```python
from build123d import *

# Parameters (mm, degrees)
BOSS_EXTRUDE1_DEPTH                   = 4
SKETCH3_R                             = 1
CUT_EXTRUDE2_DEPTH                    = 96.498691091
SKETCH4_R                             = 1
CUT_EXTRUDE3_DEPTH                    = 88.017239671
TAP_DRILL_FOR_M3X0_5_TAP2_D           = 2.5
TAP_DRILL_FOR_M3X0_5_TAP2_CSINK_D     = 2.55
TAP_DRILL_FOR_M3X0_5_TAP2_CSINK_ANGLE = 90
M3_CLEARANCE_HOLE2_D                  = 3.6
M3_CLEARANCE_HOLE2_CSINK_D            = 3.65
M3_CLEARANCE_HOLE2_CSINK_ANGLE        = 90
FILLET1_R                             = 2
CHAMFER1_SIZE                         = 2
FILLET2_R                             = 2


# Read off the part's stored shape, not the designer's step: Tap Drill for M3x0.5 Tap4, Tap Drill for M3x0.5 Tap5
with BuildPart() as part:
    # Sketch1 → Boss-Extrude1 (new, symmetric)
    with BuildSketch(Plane(origin=(0, 0, 0), x_dir=(1, 0, 0), z_dir=(0, 1, 0))):
        with BuildLine():
            Line((0, 8), (-10, 8))
            Line((-10, 8), (-10, -8))
            Line((-10, -8), (0, -8))
            Line((0, -8), (0, -14))
            Line((0, -14), (70, -26))
            Line((70, -26), (80, -26))
            Line((80, -26), (80, -20))
            Line((80, -20), (70, -20))
            Line((70, -20), (66.619956187, -19.345797972))
            ThreePointArc((66.619956187, -19.345797972), (65.457260938, -18.655013265), (65, -17.38223827))
            Line((65, -17.38223827), (65, 17.38223827))
            ThreePointArc((65, 17.38223827), (65.457260938, 18.655013265), (66.619956187, 19.345797972))
            Line((66.619956187, 19.345797972), (70, 20))
            Line((70, 20), (80, 20))
            Line((80, 20), (80, 26))
            Line((80, 26), (70, 26))
            Line((70, 26), (0, 14))
            Line((0, 14), (0, 8))
        make_face()
        with BuildLine():
            Line((8, 6.349980206), (8, -6.349980206))
            ThreePointArc((8, -6.349980206), (8.457260938, -7.622755201), (9.619956187, -8.313539907))
            Line((9.619956187, -8.313539907), (54.619956187, -17.023217326))
            ThreePointArc((54.619956187, -17.023217326), (56.272774995, -16.602396687), (57, -15.059657625))
            Line((57, -15.059657625), (57, 15.059657625))
            ThreePointArc((57, 15.059657625), (56.272774995, 16.602396687), (54.619956187, 17.023217326))
            Line((54.619956187, 17.023217326), (9.619956187, 8.313539907))
            ThreePointArc((9.619956187, 8.313539907), (8.457260938, 7.622755201), (8, 6.349980206))
        make_face(mode=Mode.SUBTRACT)
    extrude(amount=BOSS_EXTRUDE1_DEPTH, both=True)

    # Sketch3 → Cut-Extrude2 (cut, through all)
    with BuildSketch(Plane.XY.offset(26)):
        with Locations((75, 0)):
            Circle(SKETCH3_R)
    extrude(amount=-CUT_EXTRUDE2_DEPTH, mode=Mode.SUBTRACT)

    # Sketch4 → Cut-Extrude3 (cut, through all)
    with BuildSketch(Plane.XY.offset(8)):
        with Locations((-7, 0)):
            Circle(SKETCH4_R)
    extrude(amount=-CUT_EXTRUDE3_DEPTH, mode=Mode.SUBTRACT)

    # Tap Drill for M3x0.5 Tap2 (through all)
    with Locations(Plane.XY.offset(8)):
        with Locations((-7, 0)):
            CounterSinkHole(TAP_DRILL_FOR_M3X0_5_TAP2_D / 2, TAP_DRILL_FOR_M3X0_5_TAP2_CSINK_D / 2, counter_sink_angle=TAP_DRILL_FOR_M3X0_5_TAP2_CSINK_ANGLE)

    # M3 Clearance Hole2 (through all)
    with Locations(Plane.XY.offset(26)):
        with Locations((75, 0)):
            CounterSinkHole(M3_CLEARANCE_HOLE2_D / 2, M3_CLEARANCE_HOLE2_CSINK_D / 2, counter_sink_angle=M3_CLEARANCE_HOLE2_CSINK_ANGLE)

    # Fillet1
    fillet1_edges = [part.edges().sort_by_distance(p)[0] for p in [
        (-10, 4, 0),
        (80, -4, -23),
        (80, -4, 23),
        (-10, -4, 0),
        (80, 4, 23),
        (80, 4, -23),
    ]]
    fillet(fillet1_edges, radius=FILLET1_R)

    # Chamfer1
    chamfer1_edges = [part.edges().sort_by_distance(p)[0] for p in [
        (0, 4, 11),
        (0, -4, 11),
        (0, -4, -11),
        (0, 4, -11),
    ]]
    chamfer(chamfer1_edges, length=CHAMFER1_SIZE)

    # Tap Drill for M3x0.5 Tap4 outline → Tap Drill for M3x0.5 Tap4 (revolve, cut)
    with BuildSketch(Plane(origin=(41.33148295, 0, 7.085397077), x_dir=(0.9856222548132666, 0, 0.1689638151108459), z_dir=(0, 1, 0))):
        Polygon((1.25, -13.773711567), (1.25, -7.206179724), (0, -7.206179724), (0, -13.798711567), (1.275, -13.798711567), align=None)
    revolve(axis=Axis((41.33148295, 0, 7.085397077), (0.1689638151108459, 0, -0.9856222548132666)), mode=Mode.SUBTRACT)

    # Tap Drill for M3x0.5 Tap5 outline → Tap Drill for M3x0.5 Tap5 (revolve, cut)
    with BuildSketch(Plane(origin=(41.33148295, 0, -7.085397077), x_dir=(0.9856222548132666, 0, -0.1689638151108459), z_dir=(0, -1, 0))):
        Polygon((1.25, -13.773711567), (1.25, -7.206546017), (0, -7.206546017), (0, -13.798711567), (1.275, -13.798711567), align=None)
    revolve(axis=Axis((41.33148295, 0, -7.085397077), (0.1689638151108459, 0, 0.9856222548132666)), mode=Mode.SUBTRACT)

    # Fillet2
    # the kernel refuses this fillet: 2 mm, written as the material it takes off along each edge
    with BuildSketch(Plane(origin=(-9.827467058, -4, 12.315291362), x_dir=(0.1689638151108459, 0, -0.9856222548132667), z_dir=(0.9856222548132667, 0, 0.16896381511084588)), Plane(origin=(-9.827467058, 4, 12.315291362), x_dir=(0, -1, 0), z_dir=(0.9856222548132667, 0, 0.16896381511084588)), Plane(origin=(81.827467058, -4, -28.027565781), x_dir=(0.16896381511084588, 0, 0.9856222548132667), z_dir=(-0.9856222548132667, 0, 0.16896381511084588)), Plane(origin=(81.827467058, 4, -28.027565781), x_dir=(0, -1, 0), z_dir=(-0.9856222548132667, 0, 0.16896381511084588))) as fillet2_piece_1:
        with BuildLine():
            CenterArc((FILLET2_R, FILLET2_R), FILLET2_R, 180, 90)
            Line((0, FILLET2_R), (-FILLET2_R * 0.02, FILLET2_R))
            Line((-FILLET2_R * 0.02, FILLET2_R), (-FILLET2_R * 0.02, -FILLET2_R * 0.02))
            Line((-FILLET2_R * 0.02, -FILLET2_R * 0.02), (FILLET2_R, -FILLET2_R * 0.02))
            Line((FILLET2_R, -FILLET2_R * 0.02), (FILLET2_R, 0))
        make_face()
    extrude(amount=92.991948658, mode=Mode.SUBTRACT)


solid = part.part
```
Geometry: final body of the model. Coordinates: model frame, mm. A direction names the side the tool comes from. Coordinates: 2 decimals unless noted, no trailing zeros. Order: outer loops, then holes, each group sorted by start corner. A loop starts at its lowest first (then second) coordinate and runs counter-clockwise, first axis right, second up. Notation, with made-up numbers: (53.25, 55) -> (89.25, 55) arc R15 ccw to (89.25, 76) -> close; hole circle Ø1 at (63.5, 35.5). An arc over 180 degrees is marked (long way). Write each question's results on one line, items separated by ' | '. Start each with the question number.
1) Cut plane D-D, the plane x = 75. State how many separate pieces and enclosed holes the cut face has, and give its area (3 significant figures).
2) Material intervals for line 1 along X through (y, z) = (0, 1.25); line 2 along Y through (x, z) = (75, -22); line 3 along X through (y, z) = (0.75, 1), sorted ascending.
3) First-contact query: pin 1 (2.5 mm diameter, centred on y = 0.5, z = 2.5, fed in from +X); pin 2 (4 mm diameter, centred on x = 40.5, y = 2, fed in from +Z); pin 3 (3 mm diameter, centred on y = 0.5, z = -10.5, fed in from -X). Flat tips, straight axial feed; report the tip coordinate or a pass-through.
4) Cut plane A-A, the plane z = -2. Output: boundary loops of the cut face in (x, y).
5) Cut plane C-C, the plane z = 10. Output: boundary loops of the cut face in (x, y).
6) Mould query, pull axis X, two halves, no side actions, for faces 1 (the flat face through (1, 3, -11)), 2 (the cylindrical face through (56.25, 0.06, 16.62)), 3 (the flat face through (32, -4, 13)). Classes: released by +X, released by -X, zero draft, split by the parting line, or undercut.
7) Set-up query: faces 4 (the cylindrical face through (65.445, 0.056, -18.64)), 5 (the flat face through (1, -3, -11)), 6 (the flat face through (1, -3, 11)). Return all of +Z, -Z, +X, -X, +Y, -Y with unobstructed straight access to the full face (end or side cutting, diameter ignored); none if empty.
8) Cut plane B-B, the plane x = -7. Output: boundary loops of the cut face in (y, z) (3 decimals).
Checks:
1) separate pieces: 4 | enclosed holes: 0 | area: 52.2 mm^2
2) line 1: -10 to -8.25, -5.75 to 8, 57 to 65 | line 2: -4 to -1.8, 1.8 to 4 | line 3: -10 to -8, -6 to 8, 57 to 65
3) pin 1: x = 65 | pin 2: z = 21.29 | pin 3: x = 0
4) outline: (-10, -2) arc R2 ccw to (-8, -4) -> (8, -4) -> (8, 4) -> (-8, 4) arc R2 ccw to (-10, 2) -> close; (57, -4) -> (65, -4) -> (65, 4) -> (57, 4) -> close; hole circle Ø2.5 at (-7, 0)
5) outline: (0, -2) -> (2, -4) -> (18.33, -4) -> (18.33, 4) -> (2, 4) -> (0, 2) -> close; (57, -4) -> (65, -4) -> (65, 4) -> (57, 4) -> close
6) face 1: released by -X | face 2: undercut | face 3: zero draft
7) face 4: +X, +Y, -Y | face 5: -Z, -X, -Y | face 6: +Z, -X, -Y
8) outline: (-4, -8) -> (-1.25, -8) -> (-1.25, 7.975) -> (-1.275, 8) -> (-4, 8) -> close; (1.25, -8) -> (4, -8) -> (4, 8) -> (1.275, 8) -> (1.25, 7.975) -> close
